Could you check a few things on this model? Use its own coordinates, in mm. Coordinates: 2 decimals unless noted, no trailing zeros. Loops run counter-clockwise (first coordinate to the right, second up) from the corner with the lowest first, then second, coordinate; pieces in that order, holes last. Notation, with made-up numbers: (87.5, -1) - (104.5, -1) arc R15 ccw to (104.5, 8) - close; hole circle Ø2 at (70.5, 20). An arc over 180 degrees is marked (long way). Use CSV: the item, a comma, the result in double quotes.
from build123d import *

# Parameters (mm, degrees)
SKETCH019_W    = 10
SKETCH019_H    = 2.7812096768
SKETCH005_W    = 10
SKETCH005_H    = 2.2955317108
CYLINDER_R     = 1.4
CYLINDER_DEPTH = 10
ARRAY001_COUNT = 3
SKETCH018_W    = 3.15
SKETCH018_H    = 2.3
SKETCH002_W    = 5
SKETCH002_H    = 6.8
ARRAY_Z_COUNT  = 6
ARRAY_Z_PITCH  = 1.6


with BuildPart() as obj1:
    # Sketch019 → Revolution008 (revolve)
    with BuildSketch(Plane.XZ):
        with Locations((5, 3.1861365492)):
            Rectangle(SKETCH019_W, SKETCH019_H)
    revolve(axis=Axis((0, 0, 0), (0, 0, 1)))


with BuildPart() as clone_of_lowerdomain001:
    # Sketch005 → Revolution004 (revolve)
    with BuildSketch(Plane.XZ):
        with Locations((5, 0.6477658554)):
            Rectangle(SKETCH005_W, SKETCH005_H)
    revolve(axis=Axis((0, 0, 0), (0, 0, 1)))


with BuildPart() as boltholes:
    # Cylinder → Cylinder (new body)
    with BuildSketch(Plane(origin=(0, 6, -1), x_dir=(1, 0, 0), z_dir=(0, 0, 1))):
        Circle(CYLINDER_R)
    extrude(amount=CYLINDER_DEPTH)

    # Array001: BoltHoles ×3 about axis
    array001_axis = Axis((0, 0, 0), (0, 0, 1))


with BuildPart() as boltholes_1:
    add(boltholes.part)
    for i in range(1, ARRAY001_COUNT):
        add(boltholes.part.rotate(array001_axis, i * 360 / ARRAY001_COUNT))


with BuildPart() as obj2:
    # Sketch018 → Revolution007 (revolve)
    with BuildSketch(Plane.XZ):
        with Locations((1.575, 5.7267413876)):
            Rectangle(SKETCH018_W, SKETCH018_H)
    revolve(axis=Axis((0, 0, 0), (0, 0, 1)))


with BuildPart() as obj3:
    # Sketch007 → Revolution006 (revolve)
    with BuildSketch(Plane.XZ):
        with BuildLine():
            ThreePointArc((1.5, 1.7955317108), (0.867020761, 2.4322916436), (0, 2.6655317108))
            Line((0, 2.6655317108), (0, 0.7955317108))
            Line((0, 0.7955317108), (1.5, 0.7955317108))
            Line((1.5, 1.7955317108), (1.5, 0.7955317108))
        make_face()
    revolve(axis=Axis((0, 0, 0), (0, 0, 1)))


with BuildPart() as obj4:
    # Sketch002 → Revolution002 (revolve)
    with BuildSketch(Plane.XZ):
        with Locations((7.5, 3.8)):
            Rectangle(SKETCH002_W, SKETCH002_H)
    revolve(axis=Axis((0, 0, 0), (0, 0, 1)))


with BuildPart() as innergroovetool:
    # Sketch001 → Revolution001 (revolve)
    with BuildSketch(Plane.XZ):
        Polygon((4, 8), (4, 6.4), (8, 6.4), (8.8, 7.2), (8, 8), align=None)
    revolve(axis=Axis((0, 0, 0), (0, 0, 1)))

    # Array Z: InnerGrooveTool ×6


with BuildPart() as innergroovetool_1:
    add(innergroovetool.part)
    with Locations(*[(0, 0, -i * ARRAY_Z_PITCH) for i in range(1, ARRAY_Z_COUNT)]):
        add(innergroovetool.part)

    # Common: intersect obj4
    add(obj4.part, mode=Mode.INTERSECT)


with BuildPart() as refine_middlecommon:
    # Sketch → Revolution (revolve)
    with BuildSketch(Plane.XZ):
        Polygon((1.2, 0.4), (8, 0.4), (8, 7.2), (2.8, 7.2), (1.2, 2.2), align=None)
    revolve(axis=Axis((0, 0, 0), (0, 0, 1)))

    # Fusion001: union InnerGrooveTool
    add(innergroovetool_1.part)

    # Cut: cut obj3
    add(obj3.part, mode=Mode.SUBTRACT)

    # Cut003: cut obj2
    add(obj2.part, mode=Mode.SUBTRACT)

    # Cut001: cut BoltHoles
    add(boltholes_1.part, mode=Mode.SUBTRACT)

    # Cut002: cut Clone of LowerDomain001
    add(clone_of_lowerdomain001.part, mode=Mode.SUBTRACT)

    # Common002: intersect obj1
    add(obj1.part, mode=Mode.INTERSECT)


solid = refine_middlecommon.part
(1) Please list where these lines run through material, in increasing order: line 1 (Y direction, x = 0, z = 3.05); line 2 (Y direction, x = -1, z = 3.4); line 3 (Z direction, x = 5, y = -7).
Computed:
line 1,"y = -8.15 to -1.47, 1.47 to 4.6, 7.4 to 8.15"
line 2,"y = -8.14 to -1.23, 1.23 to 5.02, 6.98 to 8.14"
line 3,"z = 2.2 to 2.6, 3.8 to 4.2"
(2) Will these pins go through, and if not, where does the flat tip stop? pin 1 (4.5 mm diameter, centred on x = 0, y = 6, fed in from -Z); pin 2 (1 mm diameter, centred on x = 4.5, z = 4, fed in from -Y).
Computed:
pin 1,"stops at z = 1.8"
pin 2,"stops at y = -7.84"
(3) Thinking about a two-plate mould opening in X: for faces 1 (the face through (-0.18, 7.39, 3.17)), 2 (the face through (3.8, -2.9, 3.2)), 3 (the face through (-2, -2, 4.577)), which applies, +X half, -X half, draft (parallel to the pull), parting line (faces both ways), or undercut?
Computed:
face 1,"undercut"
face 2,"undercut"
face 3,"draft"
(4) Suppose I cut it at B-B (z = 3.75). Write out the boundary of the cut face in (x, y), plus the area to 3 significant figures.
Computed:
outline,"circle Ø17.1 at (0, 0); hole circle Ø2.8 at (-5.2, -3); hole circle Ø3.39 at (0, 0); hole circle Ø2.8 at (0, 6); hole circle Ø2.8 at (5.2, -3)"
area,"202 mm²"
(5) Suppose I cut it at A-A (x = 0). State how many separate pieces and enclosed holes the cut face has, plus the area to 3 significant figures.
Computed:
separate pieces,"3"
enclosed holes,"0"
area,"30.6 mm²"
